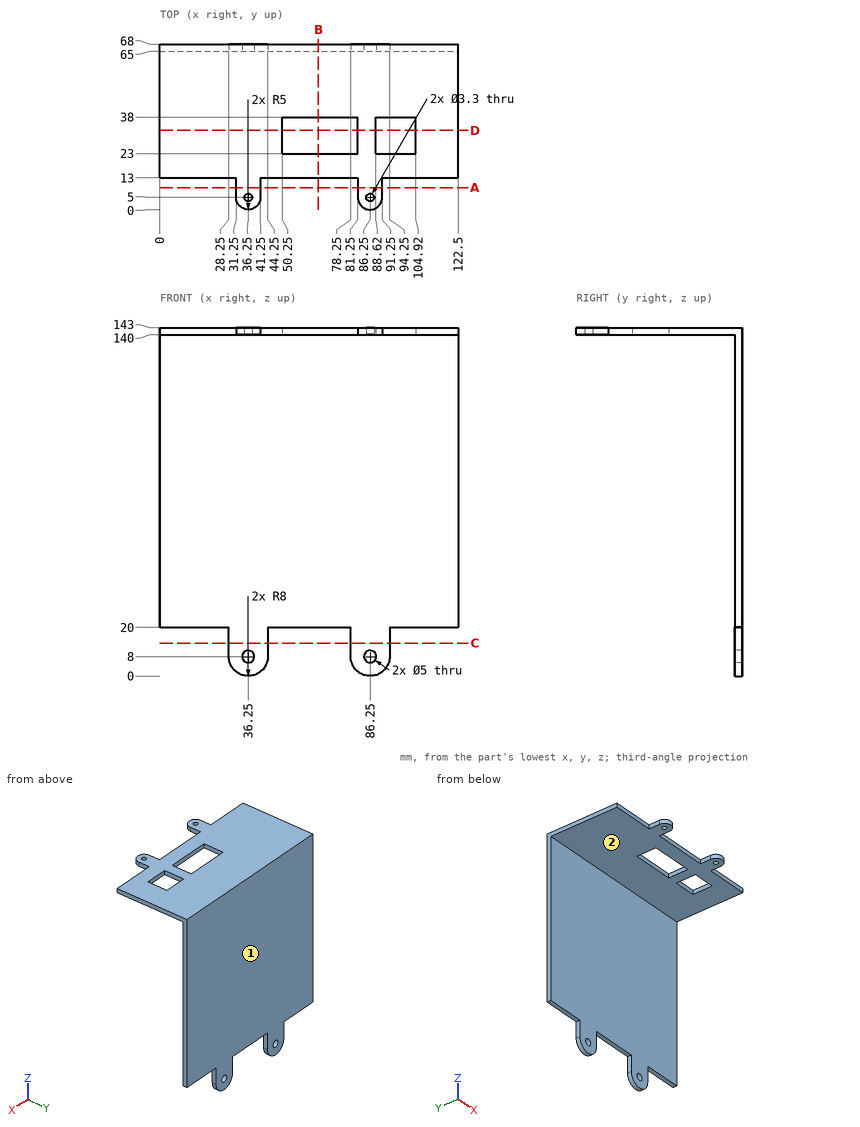
Input: dimensioned drawing with shaded views. Units: mm. Origin: part minimum x, y, z. A direction names the side the tool comes from. Coordinates: 2 decimals unless noted, no trailing zeros. Write each loop counter-clockwise with the first axis right and the second up, starting at its lowest first coordinate (ties: lowest second). Pieces come first, ordered by that corner, then holes. Notation, with made-up numbers: (65, 79) -> (101, 79) arc R18 ccw to (101, 111) -> close; hole circle Ø6 at (-25, -37.75). An arc over 180 degrees is marked (long way). Return JSON: item names as keys, results as strings. Group by question number.
1) Section query B-B, the plane x = 65. Return loops of the section in (y, z).
2) Section query D-D, the plane y = 32.5. Return loops of the section in (x, z).
3) Ray query, line 1 along Z through (x, y) = (86, 67); line 2 along Y through (x, z) = (86, 142); line 3 along Y through (x, z) = (17.5, 86.5). Return the intervals inside material, ascending.
4) Set-up query: the marked faces 1 and 2. Return all of +Z, -Z, +X, -X, +Y, -Y with unobstructed straight access to the full face (end or side cutting, diameter ignored); none if empty.
5) Section query A-A, the plane y = 9. Return loops of the section in (x, z), plus the area to 3 significant figures.
6) Contact query for flat-ended pins moving along their axis: P1, Ø2, axis at x = 15.5, z = 62, coming from the -Y side; P2, Ø2, axis at x = 103, y = 50, coming from the -Z side; P3, Ø3.5, axis at x = 103, y = 67, coming from the -Z side. Output: stop coordinate, or through.
7) Section query C-C, the plane z = 13.5. Return loops of the section in (x, y), plus the area to 3 significant figures.
From the geometry:
{
 "1": {"outline": "(13, 140) -> (23, 140) -> (23, 143) -> (13, 143) -> close; (38, 140) -> (65, 140) -> (65, 20) -> (68, 20) -> (68, 143) -> (38, 143) -> close"},
 "2": {"outline": "(0, 140) -> (50.25, 140) -> (50.25, 143) -> (0, 143) -> close; (81.25, 140) -> (88.62, 140) -> (88.62, 143) -> (81.25, 143) -> close; (104.92, 140) -> (122.5, 140) -> (122.5, 143) -> (104.92, 143) -> close"},
 "3": {"line 1": "0 to 5.51, 10.49 to 143", "line 2": "0.01 to 3.37, 6.63 to 68", "line 3": "65 to 68"},
 "4": {"face 1": "+Z, -Z, +X, -X, +Y", "face 2": "-Z, +X, -X, -Y"},
 "5": {"outline": "(31.25, 140) -> (41.25, 140) -> (41.25, 143) -> (31.25, 143) -> close; (81.25, 140) -> (91.25, 140) -> (91.25, 143) -> (81.25, 143) -> close", "area": "60.0 mm²"},
 "6": {"P1": "y = 65", "P2": "z = 140", "P3": "z = 20"},
 "7": {"outline": "(28.25, 65) -> (44.25, 65) -> (44.25, 68) -> (28.25, 68) -> close; (78.25, 65) -> (94.25, 65) -> (94.25, 68) -> (78.25, 68) -> close", "area": "96.0 mm²"}
}
